Source: CAD feature listing. Evaluate the final solid. Frame: model axes, mm. Face numbers are marked on the shaded views. A direction names the side the tool comes from. Give positions to 0.01 mm unless a question says otherwise; leave off trailing zeros. Order: outer loops, then holes, each group sorted by start corner. A loop starts at its lowest first (then second) coordinate and runs counter-clockwise, first axis right, second up. Notation, with made-up numbers: M -32,-25.75 L 11,-25.75 A25 ccw 11,-1.75 Z; hole C 62.25,71 d2. An arc over 180 degrees is marked long. Return JSON: item names as keys, results as strings.
from build123d import *

# Parameters (mm, degrees)
F0_W     = 510
F0_H     = 580
F1_DEPTH = 25
F2_W     = 510
F2_H     = 130
F3_DEPTH = 470
F4_W     = 72.998022
F4_H     = 60.818438
F4_W_2   = 79.273899
F4_W_3   = 65.625256
F4_H_2   = 59.164775
F4_W_4   = 61.082054
F5_DEPTH = 500


with BuildPart() as f1:
    # F0 (on Front) → F1 (new body)
    with BuildSketch(Plane.XZ):
        with Locations((-11.220857, 106.207754)):
            Rectangle(F0_W, F0_H)
    extrude(amount=F1_DEPTH)

    # F2 (on face) → F3 (join)
    with BuildSketch(Plane.XZ.offset(25)):
        with Locations((-11.220857, 331.207754)):
            Rectangle(F2_W, F2_H)
    extrude(amount=F3_DEPTH)

    # F4 (on face) → F5 (join)
    with BuildSketch(Plane(origin=(0, 0, 0), x_dir=(-1, 0, 0), z_dir=(0, 1, 0))):
        with Locations((-207.280132, 365.798535)):
            Rectangle(F4_W, F4_H)
        with Locations((226.583907, 365.798535)):
            Rectangle(F4_W_2, F4_H)
        with Locations((-210.966515, -154.209858)):
            Rectangle(F4_W_3, F4_H_2)
        with Locations((235.67983, -154.209858)):
            Rectangle(F4_W_4, F4_H_2)
    extrude(amount=F5_DEPTH)


solid = f1.part
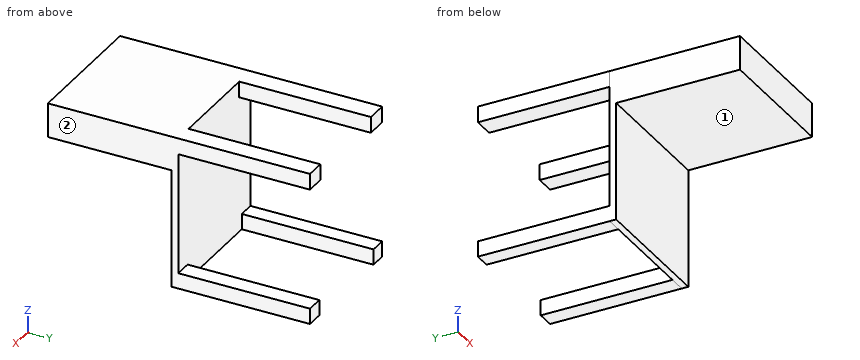
1. Section query B-B (x = -7). Return loops of the section in (y, z), then the cut area to 3 significant figures.
Evaluation:
{"outline": "M -495,266.21 L -25,266.21 L -25,-183.79 L 0,-183.79 L 0,396.21 L -495,396.21 Z", "area": "75,600 mm^2"}
2. Ray query, probe 1 along Z at (x, y) = (196.5, 384); probe 2 along Y at (x, z) = (-115.5, 349); probe 3 along Y at (x, z) = (-237, 158). Return the intervals inside material, ascending.
Evaluation:
{"probe 1": "z = -183.79 to -124.63, 335.39 to 396.21", "probe 2": "y = -495 to 0", "probe 3": "y = -25 to 0"}
3. Section query A-A (y = 35). Return loops of the section in (x, z), then the cut area to 3 significant figures.
Evaluation:
{"outline": "M -266.22,-183.79 L -205.14,-183.79 L -205.14,-124.63 L -266.22,-124.63 Z; M -266.22,335.39 L -186.95,335.39 L -186.95,396.21 L -266.22,396.21 Z; M 170.78,335.39 L 243.78,335.39 L 243.78,396.21 L 170.78,396.21 Z; M 178.15,-183.79 L 243.78,-183.79 L 243.78,-124.63 L 178.15,-124.63 Z", "area": "16,800 mm^2"}
4. Section query D-D (x = -226.5). Return loops of the section in (y, z), then the cut area to 3 significant figures.
Evaluation:
{"outline": "M -495,266.21 L -25,266.21 L -25,-183.79 L 500,-183.79 L 500,-124.63 L 0,-124.63 L 0,335.39 L 500,335.39 L 500,396.21 L -495,396.21 Z", "area": "136,000 mm^2"}
5. First-contact query: pin 1 (10 mm diameter, centred on x = 2, z = 56.5, fed in from +Y). Flat tip, straight axial feed; report the tip coordinate or a pass-through.
Evaluation:
{"pin 1": "stops at y = 0"}
6. Section query C-C (z = 80). Return loops of the section in (x, y).
Evaluation:
{"outline": "M -266.22,-25 L 243.78,-25 L 243.78,0 L -266.22,0 Z"}
7. Set-up query: the marked faces 1 and 2. Return all of +Z, -Z, +X, -X, +Y, -Y with unobstructed straight access to the full face (end or side cutting, diameter ignored); none if empty.
Evaluation:
{"face 1": "-Z, +X, -X, -Y", "face 2": "+Z, -Z, +X, +Y, -Y"}
